Autodesk Inventor part; units mm, degrees
ref_plane "YZ Plane" through (0, 0, 0) normal (1, 0, 0) x (0, 1, 0)
ref_plane "XZ Plane" through (0, 0, 0) normal (0, 1, 0) x (-1, 0, 0)
ref_plane "XY Plane" through (0, 0, 0) normal (0, 0, 1) x (1, 0, 0)
sketch "Sketch1" plane through (0, 0, 0) normal (0, 0, 1) x (1, 0, 0)
  line L0 (0, 0) -> (66.903, 0)
  line L1 (66.903, 0) -> (66.903, 38.1)
  line L2 (66.903, 38.1) -> (0, 38.1)
  line L3 (0, 38.1) -> (0, 0)
  dimension "d0" = 66.903
  dimension "d1" = 38.1
extrude "Extrusion1" add sketch "Sketch1" along normal blind 88.9
sketch "Sketch2" plane through (0, 38.1, 0) normal (0, 1, 0) x (1, 0, 0)
  line L0 (0, -88.9) -> (66.903, -88.9)
  line L1 (0, -88.9) -> (38.1, -88.9)
  line L2 (38.1, -88.9) -> (38.1, -38.1)
  line L3 (38.1, -38.1) -> (0, -38.1)
  line L4 (0, -38.1) -> (0, -88.9)
  point P0 (0, 0)
  dimension "d4" = 38.1
  dimension "d5" = 50.8
extrude "Extrusion2" cut sketch "Sketch2" against normal through all
sketch "Sketch3" plane through (0, 0, 0) normal (0, 0, -1) x (-1, 0, 0)
  line L0 (-66.903, 38.1) -> (0, 38.1)
  line L1 (-66.903, 38.1) -> (-88.9, 0)
  line L2 (-88.9, 0) -> (-66.903, 0)
  line L3 (-66.903, 0) -> (-66.903, 38.1)
  point P0 (0, 0)
  dimension "d8" = 60
extrude "Extrusion3" add sketch "Sketch3" against normal blind 88.9
properties part number "BO04" material "Wood (Oak)"
Read the model definition and answer for the solid it produces. Units are mm, in the model's axes. A direction names the side the tool comes from. Give positions to 0.01 mm unless a question says otherwise; leave off trailing zeros. Write each loop counter-clockwise with the first axis right and the second up, starting at its lowest first coordinate (ties: lowest second). Pieces come first, ordered by that corner, then holes. Notation, with made-up numbers: (52, 62.25) - (81, 62.25) arc R30 ccw to (81, 101.25) - close; hole circle Ø3 at (25.25, 34). An arc over 180 degrees is marked (long way). Use CSV: the item, a comma, the result in double quotes. Start each with the question number.
Item 1: The part is cut by section D-D, the plane y = 5. Give the vertices of the cut face in (x, z).
Item 2: Flat-ended cylindrical pins translate along their axes: P1, Ø6, axis at y = 32, z = 41, coming from the +X side; P2, Ø5, axis at x = 27.5, y = 13, coming from the -Z side; P3, Ø8, axis at y = 22.5, z = 74, coming from the -X side; P4, Ø5, axis at y = 14, z = 65, coming from the +X side. Find the tip coordinate at first contact, or state that the pin passes through.
Item 3: The part is cut by section A-A, the plane y = 10.5. Give the vertices of the cut face in (x, z).
Item 4: The part is cut by section B-B, the plane x = 20.5. Give the vertices of the cut face in (y, z).
Item 5: For faces 1 (the flat face through (55, 0, 34)), 2 (the flat face through (19, 19, 38.1)), determine the directions among +Z, -Z, +X, -X, +Y, -Y from which every point of the face is accessible in a straight line to the end or side of a thin tool.
Item 6: The part is cut by section C-C, the plane z = 17. Give the vertices of the cut face in (x, y), and give its area (3 significant figures).
Item 7: Consider line 1 (Z direction, x = 20.5, y = 4.5); line 2 (X direction, y = 8.5, z = 15); line 3 (X direction, y = 7, z = 27.5). Determine where each line is inside the solid, lowest interval first.
Taken from the geometry:
1,outline,"(0, 0) - (86.01, 0) - (86.01, 88.9) - (38.1, 88.9) - (38.1, 38.1) - (0, 38.1) - close"
2,P1,"x = 72.16"
2,P2,"z = 0"
2,P3,"x = 38.1"
2,P4,"x = 82.26"
3,outline,"(0, 0) - (82.84, 0) - (82.84, 88.9) - (38.1, 88.9) - (38.1, 38.1) - (0, 38.1) - close"
4,outline,"(0, 0) - (38.1, 0) - (38.1, 38.1) - (0, 38.1) - close"
5,face 1,"+Z, -Z, +X, -X, -Y"
5,face 2,"+Z, -X, +Y, -Y"
6,outline,"(0, 0) - (88.9, 0) - (66.9, 38.1) - (0, 38.1) - close"
6,area,"2,970 mm2"
7,line 1,"0 to 38.1"
7,line 2,"0 to 83.99"
7,line 3,"0 to 84.86"
